The model under review builds one solid part; all positions refer to its coordinate system, in mm. Coordinates: 2 decimals unless noted, no trailing zeros. Write each loop counter-clockwise with the first axis right and the second up, starting at its lowest first coordinate (ties: lowest second). Pieces come first, ordered by that corner, then holes. Notation, with made-up numbers: (61, 45.5) -> (99, 45.5) arc R8 cw to (99, 58.5) -> close; hole circle Ø3 at (2, -18). An arc over 180 degrees is marked (long way). Write each question's results on one line, items separated by ' | '.
```python
from build123d import *

# Parameters (mm, degrees)
SKETCH1_R           = 45
BOSS_EXTRUDE1_DEPTH = 454.226626
SKETCH2_R           = 15.646938019
CUT_EXTRUDE1_DEPTH  = 459.663087426
CHAMFER1_SIZE       = 0.507777


with BuildPart() as part:
    # Sketch1 → Boss-Extrude1 (new body)
    with BuildSketch(Plane(origin=(0, 0, 0), x_dir=(1, 0, 0), z_dir=(0, 1, 0))):
        with Locations(Location((0, 0, 0), (0, 0, 270))):
            Circle(SKETCH1_R)
    extrude(amount=BOSS_EXTRUDE1_DEPTH)

    # Sketch2 → Cut-Extrude1 (cut, through all)
    with BuildSketch(Plane(origin=(0, 0, 0), x_dir=(1, 0, 0), z_dir=(0, 1, 0))):
        with Locations(Location((0, 0, 0), (0, 0, 270))):
            Circle(SKETCH2_R)
    extrude(amount=CUT_EXTRUDE1_DEPTH, mode=Mode.SUBTRACT)

    # Chamfer1
    chamfer1_edges = [part.edges().sort_by_distance(p)[0] for p in [
        (0, 0, -45),
        (0, 454.226626, -45),
    ]]
    chamfer(chamfer1_edges, length=CHAMFER1_SIZE)


solid = part.part
```
Q1. For line 1 (X direction, y = 404, z = -1.5) (3 decimals); line 2 (Z direction, x = -12, y = 198); line 3 (X direction, y = 305, z = 7), list the stretches that pass through material, from the lowest coordinate up. Write a range as from..to.
Solution:
line 1: -44.975..-15.575, 15.575..44.975 | line 2: -43.37..-10.04, 10.04..43.37 | line 3: -44.45..-13.99, 13.99..44.45
Q2. Add section C-C (y = 356.5). Write out the cut boundary in (x, z).
Solution:
outline: circle Ø90 at (0, 0); hole circle Ø31.29 at (0, 0)
Q3. Clearance check with flat-ended pins moving along their axes: P1, Ø12, axis at x = -36, y = 219.5, coming from the -Z side; P2, Ø6, axis at x = -3.5, y = 374, coming from the -Z side; P3, Ø1.5, axis at y = 244.5, z = -10, coming from the -X side. State where each tip first meets the part, or that it passes through.
Solution:
P1: z = -33.54 | P2: z = -45 | P3: x = -44.04
Q4. Add section A-A (x = 0). Write out the cut boundary in (y, z), plus the area to 3 significant figures.
Solution:
outline: (0, -44.49) -> (0.51, -45) -> (453.72, -45) -> (454.23, -44.49) -> (454.23, -15.65) -> (0, -15.65) -> close; (0, 15.65) -> (454.23, 15.65) -> (454.23, 44.49) -> (453.72, 45) -> (0.51, 45) -> (0, 44.49) -> close | area: 26,700 mm²
Q5. Draft analysis for pull direction Z (two halves, no side actions). For faces 1 (the flat face through (1, 0, 19)), 2 (the cylindrical face through (-9.52, 223.93, -12.42)), 3 (the cylindrical face through (-17.235, 223.941, 41.569)), state which applies: pulls with the +Z half, pulls with the -Z half, needs draft (parallel to the pull), parting line crosses it, or undercut.
Solution:
face 1: needs draft | face 2: undercut | face 3: parting line crosses it
Q6. Add section B-B (z = 0). Write out the cut boundary in (x, y), plus the area to 3 significant figures.
Solution:
outline: (-45, 0.51) -> (-44.49, 0) -> (-15.65, 0) -> (-15.65, 454.23) -> (-44.49, 454.23) -> (-45, 453.72) -> close; (15.65, 0) -> (44.49, 0) -> (45, 0.51) -> (45, 453.72) -> (44.49, 454.23) -> (15.65, 454.23) -> close | area: 26,700 mm²
